Read the model definition and answer for the solid it produces. Units are mm, in the model's axes. Coordinates: 2 decimals unless noted, no trailing zeros. Loops run counter-clockwise (first coordinate to the right, second up) from the corner with the lowest first, then second, coordinate; pieces in that order, holes last.
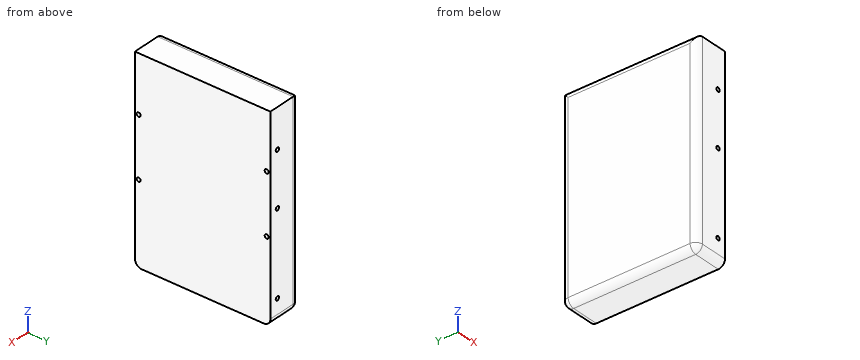
Solid Edge part; units mm, degrees
sketch "Sketch1" plane through (0, 0, 0) normal (-1, 0, 0) x (0, -1, 0)
  line L0 (-50.4025, -73.375) -> (50.4025, -73.375)
  line L1 (50.4025, -73.375) -> (50.4025, 73.375)
  line L2 (50.4025, 73.375) -> (-50.4025, 73.375)
  line L3 (-50.4025, 73.375) -> (-50.4025, -73.375)
extrude "Protrusion1" add sketch "Sketch1" along normal blind 25.55
sketch "Sketch2" plane through (-12.775, 50.4025, 0) normal (0, 1, 0) x (0, 0, -1)
  circle A0 centre (-44.225, -6.425) radius 1.5
  circle A1 centre (-4.125, -6.425) radius 1.5
  circle A2 centre (57.375, -6.425) radius 1.5
extrude "Cutout1" cut sketch "Sketch2" along normal mid plane 330
sketch "Sketch3" plane through (0, 0, 0) normal (1, 0, 0) x (0, 0, -1)
  circle A0 centre (-31.405, 47.6525) radius 1.5
  circle A1 centre (13.045, 47.6525) radius 1.5
  circle A2 centre (-31.405, -47.6525) radius 1.5
  circle A3 centre (13.045, -47.6525) radius 1.5
extrude "Cutout2" cut sketch "Sketch3" against normal blind 20
fillet "Round_6" radius 5 6 edges at (-25.55, 0, 73.375) (-25.55, -50.4025, 0) (-25.55, 0, -73.375) (-25.55, 50.4025, 0) (-12.775, 50.4025, -73.375) (-12.775, -50.4025, -73.375)
Q1. A cutting plane is placed at B-B (x = -23). Give the vertices of the cut face in (y, z) (1 decimal), then the cut area to 3 significant figures.
Findings below:
outline: (-49.8, -68.4) arc R4.4 ccw to (-45.4, -72.7) - (45.4, -72.7) arc R4.4 ccw to (49.8, -68.4) - (49.8, 72.7) - (-49.8, 72.7) - close
area: 14,500 mm2
Q2. Straight lines are drawn through the part: probe 1 along Z at (x, y) = (-6.35, -2) (3 decimals); probe 2 along Y at (x, z) = (-6, 31); probe 3 along X at (y, z) = (-45.5, -66). For each, find the intervals that lie inside material, in ascending order.
Findings below:
probe 1: z = -73.375 to -58.875, -55.875 to 2.625, 5.625 to 42.725, 45.725 to 73.375
probe 2: y = -50.4 to -49.1, -46.21 to 46.21, 49.1 to 50.4
probe 3: x = -25.55 to 0
Q3. A cutting plane is placed at A-A (x = -6.35). Give the vertices of the cut face in (y, z) (1 decimal), then the cut area to 3 significant figures.
Findings below:
outline: (-50.4, -68.4) arc R5 ccw to (-45.4, -73.4) - (45.4, -73.4) arc R5 ccw to (50.4, -68.4) - (50.4, -58.9) - (-50.4, -58.9) - close; (-50.4, -55.9) - (50.4, -55.9) - (50.4, 2.6) - (-50.4, 2.6) - close; (-50.4, 5.6) - (50.4, 5.6) - (50.4, 42.7) - (-50.4, 42.7) - close; (-50.4, 45.7) - (50.4, 45.7) - (50.4, 73.4) - (-50.4, 73.4) - close; hole circle Ø3 at (-47.7, -13); hole circle Ø3 at (-47.7, 31.4); hole circle Ø3 at (47.7, -13); hole circle Ø3 at (47.7, 31.4)
area: 13,800 mm2
Q4. Flat-ended cylindrical pins translate along their axes: pin 1 Ø1.5 at (y, z) = (47, 31.5) entering from +X; pin 2 Ø2.5 at (x, z) = (-6.35, -57.375) entering from -Y; pin 3 Ø4 at (y, z) = (47.65, -13.04) entering from -X. Find the tip coordinate at first contact, or state that the pin passes through.
Findings below:
pin 1: stops at x = -20
pin 2: passes through
pin 3: stops at x = -25.54
